```python
from build123d import *

# Parameters (mm, degrees)
CROQUIS1_W                                           = 150
CROQUIS1_H                                           = 150
SALIENTE_EXTRUIR1_DEPTH                              = 5
CROQUIS2_W                                           = 72
CROQUIS2_H                                           = 102
CORTAR_EXTRUIR1_DEPTH                                = 3
CROQUIS3_W                                           = 5
CROQUIS3_H                                           = 75
CORTAR_EXTRUIR2_DEPTH                                = 10
REDONDEO1_R                                          = 10
REDONDEO3_R                                          = 5
REFRENTADO_PARA_TORNILLO_CON_CABEZA_TRON_D           = 3.2639
REFRENTADO_PARA_TORNILLO_CON_CABEZA_TRON_DEPTH       = 50
REFRENTADO_PARA_TORNILLO_CON_CABEZA_TRON_CBORE_D     = 6.35
REFRENTADO_PARA_TORNILLO_CON_CABEZA_TRON_CBORE_DEPTH = 2.032
REFRENTADO_PARA_TORNILLO_CON_CABEZA_TRON_TIP         = 0.980574487


with BuildPart() as part:
    # Croquis1 → Saliente-Extruir1 (new body)
    with BuildSketch(Plane.XY):
        Rectangle(CROQUIS1_W, CROQUIS1_H)
    extrude(amount=SALIENTE_EXTRUIR1_DEPTH)

    # Croquis2 → Cortar-Extruir1 (cut)
    with BuildSketch(Plane.XY.offset(5)):
        Rectangle(CROQUIS2_W, CROQUIS2_H)
    extrude(amount=-CORTAR_EXTRUIR1_DEPTH, mode=Mode.SUBTRACT)

    # Croquis3 → Cortar-Extruir2 (cut)
    with BuildSketch(Plane.XY.offset(5)):
        Rectangle(CROQUIS3_W, CROQUIS3_H)
    extrude(amount=-CORTAR_EXTRUIR2_DEPTH, mode=Mode.SUBTRACT)

    # Redondeo1
    redondeo1_edges = [part.edges().sort_by_distance(p)[0] for p in [
        (75, -75, 2.5),
        (-75, -75, 2.5),
        (-75, 75, 2.5),
        (75, 75, 2.5),
    ]]
    fillet(redondeo1_edges, radius=REDONDEO1_R)

    # Redondeo3
    redondeo3_edges = [part.edges().sort_by_distance(p)[0] for p in [
        (72.071067812, 72.071067812, 5),
        (75, 0, 5),
        (72.071067812, -72.071067812, 5),
        (0, -75, 5),
        (-72.071067812, -72.071067812, 5),
        (-75, 0, 5),
        (-72.071067812, 72.071067812, 5),
        (0, 75, 5),
    ]]
    fillet(redondeo3_edges, radius=REDONDEO3_R - 0.0001)  # a hair under: the kernel refuses the full size

    # Refrentado para tornillo con cabeza troncocónica de #41
    with Locations(Plane.XY.offset(5)):
        with Locations((-70, 70), (-70, -70), (70, -70), (70, 70)):
            CounterBoreHole(REFRENTADO_PARA_TORNILLO_CON_CABEZA_TRON_D / 2, REFRENTADO_PARA_TORNILLO_CON_CABEZA_TRON_CBORE_D / 2, REFRENTADO_PARA_TORNILLO_CON_CABEZA_TRON_CBORE_DEPTH, depth=REFRENTADO_PARA_TORNILLO_CON_CABEZA_TRON_DEPTH)
            with Locations((0, 0, -(REFRENTADO_PARA_TORNILLO_CON_CABEZA_TRON_DEPTH + REFRENTADO_PARA_TORNILLO_CON_CABEZA_TRON_TIP / 2))):  # 118° drill point
                Cone(0, REFRENTADO_PARA_TORNILLO_CON_CABEZA_TRON_D / 2, REFRENTADO_PARA_TORNILLO_CON_CABEZA_TRON_TIP, mode=Mode.SUBTRACT)


solid = part.part
```
Work out the finished part from the listing and answer in its coordinate system (mm). A direction names the side the tool comes from. Give positions to 0.01 mm unless a question says otherwise; leave off trailing zeros. Return JSON: item names as keys, results as strings.
1) A tool of negligible diameter and unlimited length cuts with its end or side. For faces 1 (the cylindrical face through (73, -1, 4)), 2 (the cylindrical face through (-67.69, -67.82, 4)), from which of +Z, -Z, +X, -X, +Y, -Y can it reach the whole face along a straight path? Write none if from no direction.
Resolved:
{"face 1": "+Z, +X, +Y, -Y", "face 2": "+Z"}
2) Straight lines are drawn through the part: line 1 along X through (y, z) = (-70, 1.85); line 2 along Y through (x, z) = (-70, 2.15); line 3 along Z through (x, y) = (30.5, 30.5). For each, find the intervals that lie inside material, in ascending order. Write a range as [from, to].
Resolved:
{"line 1": "[-73.25, -71.63], [-68.37, 68.37], [71.63, 73.25]", "line 2": "[-73.09, -71.63], [-68.37, 68.37], [71.63, 73.09]", "line 3": "[0, 2]"}
3) For a pull along Z with two mould halves and no side action, classify faces 3 (the cylindrical face through (-1, -73, 4)), 4 (the cylindrical face through (-68.705, -70.993, 1.463)), 5 (the flat face through (16, 1, 0)) as +Z half, -Z half, draft (parallel to the pull), parting line (faces both ways), or undercut.
Resolved:
{"face 3": "+Z half", "face 4": "draft", "face 5": "-Z half"}
4) Each of these flat-tipped pins is pushed along its axis until it touches: pin 1 (0.9 mm diameter, centred on y = -12, z = 4, fed in from -X); pin 2 (1 mm diameter, centred on x = -30, y = -4.5, fed in from +Z); pin 3 (1.5 mm diameter, centred on x = -8.5, z = 3, fed in from +Y). Where does it stop, or does it pass through?
Resolved:
{"pin 1": "x = -73.52", "pin 2": "z = 2", "pin 3": "y = 74.47"}
